from build123d import *

# Parameters (mm, degrees)
ESBO_O1_W                = 108
ESBO_O1_H                = 50
RESSALTO_EXTRUS_O1_DEPTH = 15
ESBO_O2_R                = 10
ESBO_O2_R_2              = 5
CORTE_EXTRUS_O2_DEPTH    = 15
ESBO_O4_R                = 15
CORTE_EXTRUS_O5_DEPTH    = 3
ESBO_O5_W                = 40
ESBO_O5_H                = 4
CORTE_EXTRUS_O6_DEPTH    = 76.106590923


with BuildPart() as part:
    # Esboço1 → Ressalto-extrusão1 (new body)
    with BuildSketch(Plane.XY):
        Rectangle(ESBO_O1_W, ESBO_O1_H)
    extrude(amount=RESSALTO_EXTRUS_O1_DEPTH)

    # Esboço2 → Corte-extrusão2 (cut)
    with BuildSketch(Plane.XY):
        Circle(ESBO_O2_R)
        with Locations((42, 15)):
            Circle(ESBO_O2_R_2)
        with Locations((-42, 15)):
            Circle(ESBO_O2_R_2)
        with Locations((42, -15)):
            Circle(ESBO_O2_R_2)
        with Locations((-42, -15)):
            Circle(ESBO_O2_R_2)
        with BuildLine():
            Line((-34, 3), (-54, 3))
            Line((-54, 3), (-54, -3))
            Line((-54, -3), (-34, -3))
            ThreePointArc((-34, -3), (-31, 0), (-34, 3))
        make_face()
    extrude(amount=CORTE_EXTRUS_O2_DEPTH, mode=Mode.SUBTRACT)

    # Esboço4 → Corte-extrusão5 (cut)
    with BuildSketch(Plane.XY.offset(15)):
        Circle(ESBO_O4_R)
    extrude(amount=-CORTE_EXTRUS_O5_DEPTH, mode=Mode.SUBTRACT)

    # Esboço5 → Corte-extrusão6 (cut, through all)
    with BuildSketch(Plane.XZ.offset(25)):
        with Locations((5, 2)):
            Rectangle(ESBO_O5_W, ESBO_O5_H)
    extrude(amount=-CORTE_EXTRUS_O6_DEPTH, mode=Mode.SUBTRACT)


solid = part.part
Build history of the part. All positions in model axes, mm. A direction names the side the tool comes from. Give positions to 0.01 mm unless a question says otherwise; leave off trailing zeros. Order: outer loops, then holes, each group sorted by start corner. A loop starts at its lowest first (then second) coordinate and runs counter-clockwise, first axis right, second up. Notation, with made-up numbers: M 48,71.25 L 105,71.25 A31 cw 105,106.25 Z; hole C 50.25,49 d7. An arc over 180 degrees is marked long. Put each result on its own line as item: value.
Item 1: Cut at C-C on z = 2. Write the cut outline in (x, y).
Results are:
outline: M -54,-25 L -15,-25 L -15,25 L -54,25 L -54,3 L -34,3 A3 cw -34,-3 L -54,-3 Z; M 25,-25 L 54,-25 L 54,25 L 25,25 Z; hole C -42,-15 d10; hole C -42,15 d10; hole C 42,-15 d10; hole C 42,15 d10
Item 2: Drop flat-ended pins along their axis: pin 1 Ø9 at (x, y) = (42, 15) entering from -Z; pin 2 Ø13 at (x, y) = (-42, 15) entering from -Z; pin 3 Ø15 at (x, y) = (-1, -3.5) entering from +Z. Give the stop position or say it passes through.
Results are:
pin 1: through
pin 2: z = 0
pin 3: z = 12
Item 3: Which spindle directions (+Z, -Z, +X, -X, +Y, -Y) get a long thin tool onto all of the face, cutting with end or side? Do faces 1 (the face through (39, 0, 0)), 2 (the face through (25, 0, 2)), 3 (the face through (3, -10, 12)). Say none if no direction does.
Results are:
face 1: -Z, +X, -X, +Y, -Y
face 2: -Z, +Y, -Y
face 3: +Z
Item 4: Cut at A-A on y = 0. Write the cut outline in (x, z), then the cut area to 3 significant figures.
Results are:
outline: M -31,0 L -15,0 L -15,4 L -10,4 L -10,12 L -15,12 L -15,15 L -31,15 Z; M 10,4 L 25,4 L 25,0 L 54,0 L 54,15 L 15,15 L 15,12 L 10,12 Z
area: 865 mm2
Item 5: Cut at D-D on y = -18. Write the cut outline in (x, z), then the cut area to 3 significant figures.
Results are:
outline: M -54,0 L -46,0 L -46,15 L -54,15 Z; M -38,0 L -15,0 L -15,4 L 25,4 L 25,0 L 38,0 L 38,15 L -38,15 Z; M 46,0 L 54,0 L 54,15 L 46,15 Z
area: 1,220 mm2
Item 6: Pull direction Y, two halves, no side cores. Call faces 4 (the face through (9, -6, 4)), 5 (the face through (-1, -25, 7)), 6 (the face through (-44, 3, 7)): +Y half, -Y half, draft (parallel to the pull), parting line (faces both ways), or undercut.
Results are:
face 4: draft
face 5: -Y half
face 6: undercut
Item 7: Cut at B-B on x = -42. Write the cut outline in (y, z), then the cut area to 3 significant figures.
Results are:
outline: M -25,0 L -20,0 L -20,15 L -25,15 Z; M -10,0 L -3,0 L -3,15 L -10,15 Z; M 3,0 L 10,0 L 10,15 L 3,15 Z; M 20,0 L 25,0 L 25,15 L 20,15 Z
area: 360 mm2
Item 8: Wall check: probe 1 along Y at (x, z) = (-42, 7); probe 2 along Y at (x, z) = (41.5, 8.5); probe 3 along X at (y, z) = (-12, 13.5). Give the ranges that are in metal, low to high.
Results are:
probe 1: -25 to -20, -10 to -3, 3 to 10, 20 to 25
probe 2: -25 to -19.97, -10.03 to 10.03, 19.97 to 25
probe 3: -54 to -46, -38 to -9, 9 to 38, 46 to 54
